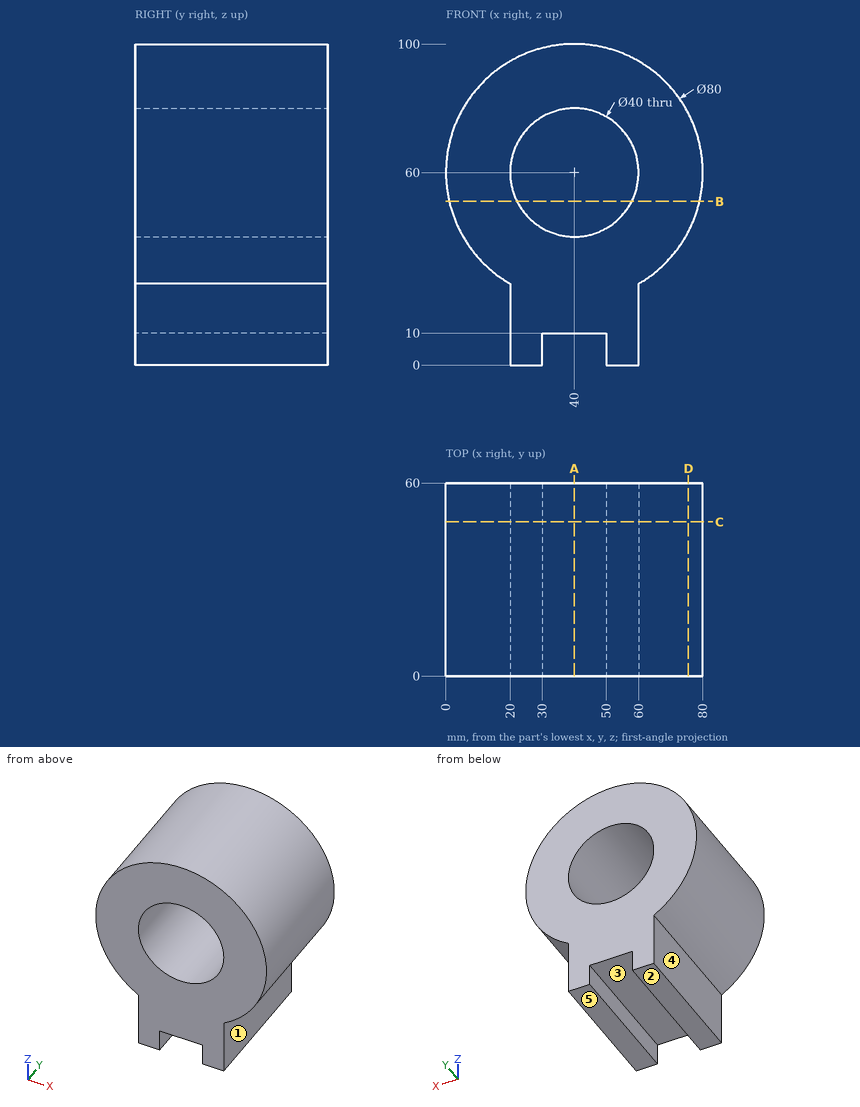
Here's the drawing with two shaded views (mm, measured from the low corner). I have some questions. A direction names the side the tool comes from. Coordinates: 2 decimals unless noted, no trailing zeros. Write each loop counter-clockwise with the first axis right and the second up, starting at its lowest first coordinate (ties: lowest second). Pieces come first, ordered by that corner, then holes. Notation, with made-up numbers: (13, 67.5) - (37, 67.5) arc R16 cw to (37, 97.5) - close; hole circle Ø1 at (-33, 33). An arc over 180 degrees is marked (long way). Return JSON: item names as keys, results as strings.
Q1. On a 3-axis mill with a long thin cutter (end or side, diameter ignored), from which of +Z, -Z, +X, -X, +Y, -Y can I reach the whole of each face in a straight line? I mean the marked faces 1 and 2. Say none if no direction works.
Computed values:
{"face 1": "-Z, +X, +Y, -Y", "face 2": "-Z, +X, -X, +Y, -Y"}
Q2. If we section it at B-B (z = 51): Please give me the cut outline in (x, y).
Computed values:
{"outline": "(1.03, 0) - (22.14, 0) - (22.14, 60) - (1.03, 60) - close; (57.86, 0) - (78.97, 0) - (78.97, 60) - (57.86, 60) - close"}
Q3. If we section it at D-D (x = 75.5): Please give me the cut outline in (y, z).
Computed values:
{"outline": "(0, 41.57) - (60, 41.57) - (60, 78.43) - (0, 78.43) - close"}
Q4. Thinking about a two-plate mould opening in X: for the marked faces 3, 4 and 5, which applies, +X half, -X half, draft (parallel to the pull), parting line (faces both ways), or undercut?
Computed values:
{"face 3": "undercut", "face 4": "-X half", "face 5": "draft"}
Q5. If we section it at C-C (y = 48): Please give me the cut outline in (x, z), then the cut area to 3 significant figures.
Computed values:
{"outline": "(20, 0) - (30, 0) - (30, 10) - (50, 10) - (50, 0) - (60, 0) - (60, 25.36) arc R40 ccw (long way) to (20, 25.36) - close; hole circle Ø40 at (40, 60)", "area": "4,440 mm2"}
Q6. I'm going to push flat-ended pins straight in: pin 1 Ø8 at (y, z) = (6.5, 34) entering from +X; pin 2 Ø11 at (y, z) = (43.5, 6) entering from +X; pin 3 Ø5 at (x, y) = (20, 45.5) entering from -Z; pin 4 Ø4 at (x, y) = (55.5, 30.5) entering from +Z. Where does each tip first touch, or does it pass through?
Computed values:
{"pin 1": "stops at x = 73.41", "pin 2": "stops at x = 60", "pin 3": "stops at z = 0", "pin 4": "stops at z = 97.65"}
Q7. Please list where these lines run through material, in increasing order: L1, parallel to Z at x = 40, y = 16; L2, parallel to X at y = 8, z = 5.5; L3, parallel to X at y = 7.5, z = 10.5. Write a range as from..to.
Computed values:
{"L1": "z = 10..40, 80..100", "L2": "x = 20..30, 50..60", "L3": "x = 20..60"}
Q8. If we section it at A-A (x = 40): Please give me the cut outline in (y, z).
Computed values:
{"outline": "(0, 10) - (60, 10) - (60, 40) - (0, 40) - close; (0, 80) - (60, 80) - (60, 100) - (0, 100) - close"}
